Part model, mm, in its own coordinate system. A direction names the side the tool comes from. Give positions to 0.01 mm unless a question says otherwise; leave off trailing zeros. Write each loop counter-clockwise with the first axis right and the second up, starting at its lowest first coordinate (ties: lowest second). Pieces come first, ordered by that corner, then holes.
from build123d import *

# Parameters (mm, degrees)
SKETCH_1_W          = 100
SKETCH_1_H          = 52
EXTRUDE_1_DEPTH     = 8.6
SKETCH_2_W          = 97
SKETCH_2_H          = 49
CUT_EXTRUDE_1_DEPTH = 3
SKETCH_3_R          = 1.1
SKETCH_3_W          = 38.632034186
SKETCH_3_H          = 7.399361665
SKETCH_3_W_2        = 5
SKETCH_3_H_2        = 5
CUT_EXTRUDE_2_DEPTH = 61.603041755
FILLET_1_R          = 2
SKETCH_4_W          = 1.5
SKETCH_4_H          = 6.8
CUT_EXTRUDE_3_DEPTH = 1
SKETCH_5_W          = 97
SKETCH_5_H          = 49
CUT_EXTRUDE_4_DEPTH = 3
EXTRUDE_2_DEPTH     = 3
FILLET_2_R          = 3
FILLET_3_R          = 2
FILLET_5_R          = 1


with BuildPart() as part:
    # 草图1 → 凸台-拉伸1 (new body)
    with BuildSketch(Plane(origin=(0, 0, 0), x_dir=(1, 0, 0), z_dir=(0, 1, 0))):
        with Locations((1.17145908, 5.982033169)):
            Rectangle(SKETCH_1_W, SKETCH_1_H)
    extrude(amount=EXTRUDE_1_DEPTH)

    # 草图2 → 切除-拉伸1 (cut)
    with BuildSketch(Plane.XZ):
        with Locations((1.17145908, -5.982033169)):
            Rectangle(SKETCH_2_W, SKETCH_2_H)
    extrude(amount=-CUT_EXTRUDE_1_DEPTH, mode=Mode.SUBTRACT)

    # 草图3 → 切除-拉伸2 (cut, through all)
    with BuildSketch(Plane.XZ.offset(-3)):
        with Locations(Location((-12.82854092, 15.517966831, 0), (0, 0, 270))):
            Circle(SKETCH_3_R)
        with Locations(Location((39.17145908, 15.517966831, 0), (0, 0, 270))):
            Circle(SKETCH_3_R)
        with Locations(Location((39.17145908, -27.482033169, 0), (0, 0, 270))):
            Circle(SKETCH_3_R)
        with Locations(Location((-12.82854092, -27.482033169, 0), (0, 0, 270))):
            Circle(SKETCH_3_R)
        with Locations((16.615396969, 13.018709543)):
            Rectangle(SKETCH_3_W, SKETCH_3_H)
        with Locations((-13.82854092, -12.482033169)):
            Rectangle(SKETCH_3_W_2, SKETCH_3_H_2)
        with Locations((23.17145908, -12.21289677)):
            Rectangle(SKETCH_3_W_2, SKETCH_3_H_2)
    extrude(amount=-CUT_EXTRUDE_2_DEPTH, mode=Mode.SUBTRACT)

    # 圆角1
    fillet_1_edges = [part.edges().sort_by_distance(p)[0] for p in [
        (20.67145908, 5.8, -14.71289677),
        (20.67145908, 5.8, -9.71289677),
        (25.67145908, 5.8, -9.71289677),
        (25.67145908, 5.8, -14.71289677),
        (-16.32854092, 5.8, -14.982033169),
        (-16.32854092, 5.8, -9.982033169),
        (-11.32854092, 5.8, -9.982033169),
        (-11.32854092, 5.8, -14.982033169),
    ]]
    fillet(fillet_1_edges, radius=FILLET_1_R)

    # 草图4 → 切除-拉伸3 (cut)
    with BuildSketch(Plane.XZ):
        with Locations((50.42145908, 0.917966831)):
            Rectangle(SKETCH_4_W, SKETCH_4_H)
    extrude(amount=-CUT_EXTRUDE_3_DEPTH, mode=Mode.SUBTRACT)

    # 草图5 → 切除-拉伸4 (cut)
    with BuildSketch(Plane(origin=(0, 8.6, 0), x_dir=(1, 0, 0), z_dir=(0, 1, 0))):
        with Locations((1.17145908, 5.982033169)):
            Rectangle(SKETCH_5_W, SKETCH_5_H)
    extrude(amount=-CUT_EXTRUDE_4_DEPTH, mode=Mode.SUBTRACT)

    # 草图7 → 凸台-拉伸2 (add, through all)
    with BuildSketch(Plane(origin=(0, 5.6, 0), x_dir=(1, 0, 0), z_dir=(0, 1, 0))):
        Polygon((-8.68854092, -18.517966831), (-8.68854092, 4.782033169), (-27.62854092, 4.782033169), (-27.62854092, 30.482033169), (-26.12854092, 30.482033169), (-26.12854092, 6.282033169), (-8.68854092, 6.282033169), (-8.68854092, 30.482033169), (-7.18854092, 30.482033169), (-7.18854092, -4.517966831), (49.67145908, -4.517966831), (49.67145908, -6.017966831), (-7.18854092, -6.017966831), (-7.18854092, -18.517966831), align=None)
        Polygon((16.97145908, 30.482033169), (16.97145908, 6.682033169), (30.17145908, 6.682033169), (30.17145908, 30.482033169), (28.67145908, 30.482033169), (28.67145908, 8.182033169), (18.47145908, 8.182033169), (18.47145908, 30.482033169), align=None)
    extrude(amount=EXTRUDE_2_DEPTH)

    # 圆角2
    fillet_2_edges = [part.edges().sort_by_distance(p)[0] for p in [
        (-48.82854092, 4.3, -31.982033169),
        (51.17145908, 4.3, -31.982033169),
        (51.17145908, 4.3, 20.017966831),
        (-48.82854092, 4.3, 20.017966831),
    ]]
    fillet(fillet_2_edges, radius=FILLET_2_R)

    # 圆角3
    fillet_3_edges = [part.edges().sort_by_distance(p)[0] for p in [
        (49.67145908, 1.5, 18.517966831),
        (49.67145908, 1.5, -30.482033169),
        (-47.32854092, 1.5, -30.482033169),
        (-47.32854092, 1.5, 18.517966831),
        (-47.32854092, 7.1, 18.517966831),
        (-47.32854092, 7.1, -30.482033169),
        (49.67145908, 7.1, -30.482033169),
        (49.67145908, 7.1, 18.517966831),
        (-8.68854092, 7.1, 18.517966831),
        (-7.18854092, 7.1, 18.517966831),
        (-7.18854092, 7.1, 6.017966831),
        (49.67145908, 7.1, 6.017966831),
        (49.67145908, 7.1, 4.517966831),
        (-7.18854092, 7.1, 4.517966831),
        (-7.18854092, 7.1, -30.482033169),
        (-8.68854092, 7.1, -30.482033169),
        (-8.68854092, 7.1, -6.282033169),
        (-26.12854092, 7.1, -6.282033169),
        (-26.12854092, 7.1, -30.482033169),
        (-27.62854092, 7.1, -30.482033169),
        (-27.62854092, 7.1, -4.782033169),
        (-8.68854092, 7.1, -4.782033169),
        (18.47145908, 7.1, -30.482033169),
        (16.97145908, 7.1, -30.482033169),
        (16.97145908, 7.1, -6.682033169),
        (30.17145908, 7.1, -6.682033169),
        (30.17145908, 7.1, -30.482033169),
        (28.67145908, 7.1, -30.482033169),
        (28.67145908, 7.1, -8.182033169),
        (18.47145908, 7.1, -8.182033169),
    ]]
    fillet(fillet_3_edges, radius=FILLET_3_R)

    # 圆角5
    fillet_5_edges = [part.edges().sort_by_distance(p)[0] for p in [
        (-2.700620124, 4.3, 16.718390375),
        (35.931414062, 4.3, 16.718390375),
        (-2.700620124, 4.3, 9.31902871),
        (35.931414062, 4.3, 9.31902871),
    ]]
    fillet(fillet_5_edges, radius=FILLET_5_R)


solid = part.part
1) Saw through at D-D (z = -18.5). Write the cut outline in (x, y), and give its area (3 significant figures).
Check result:
outline: (-48.83, 0) - (-47.33, 0) - (-47.33, 3) - (49.67, 3) - (49.67, 0) - (51.17, 0) - (51.17, 8.6) - (49.67, 8.6) - (49.67, 5.6) - (30.17, 5.6) - (30.17, 8.6) - (28.67, 8.6) - (28.67, 5.6) - (18.47, 5.6) - (18.47, 8.6) - (16.97, 8.6) - (16.97, 5.6) - (-7.19, 5.6) - (-7.19, 8.6) - (-8.69, 8.6) - (-8.69, 5.6) - (-26.13, 5.6) - (-26.13, 8.6) - (-27.63, 8.6) - (-27.63, 5.6) - (-47.33, 5.6) - (-47.33, 8.6) - (-48.83, 8.6) - close
area: 296 mm2
2) Saw through at C-C (y = 7.5). State how many separate pieces and enclosed holes the cut face has, and give its area (3 significant figures).
Check result:
separate pieces: 1
enclosed holes: 5
area: 767 mm2
3) Saw through at A-A (z = 0.5). Write the cut outline in (x, y), and give its area (3 significant figures).
Check result:
outline: (-48.83, 0) - (-47.33, 0) - (-47.33, 3) - (49.67, 3) - (49.67, 1) - (51.17, 1) - (51.17, 8.6) - (49.67, 8.6) - (49.67, 5.6) - (-7.19, 5.6) - (-7.19, 8.6) - (-8.69, 8.6) - (-8.69, 5.6) - (-47.33, 5.6) - (-47.33, 8.6) - (-48.83, 8.6) - close
area: 281 mm2
4) Saw through at B-B (x = -20.5). Write the cut outline in (y, z).
Check result:
outline: (0, -31.98) - (8.6, -31.98) - (8.6, -30.48) - (5.6, -30.48) - (5.6, -6.28) - (8.6, -6.28) - (8.6, -4.78) - (5.6, -4.78) - (5.6, 18.52) - (8.6, 18.52) - (8.6, 20.02) - (0, 20.02) - (0, 18.52) - (3, 18.52) - (3, -30.48) - (0, -30.48) - close
5) Mould opens along Z. For faces 1 (the cylindrical face through (28.1, 7.12, -8.78)), 2 (the cylindrical face through (50.27, 4.36, 19.16)), 3 (the flat face through (1, 4, -31.982)) say: +Z half, -Z half, draft (parallel to the pull), parting line (faces both ways), or undercut.
Check result:
face 1: undercut
face 2: +Z half
face 3: -Z half
6) Drill centre lines: L1, parallel to X at y = 7.25, z = 13; L2, parallel to Z at x = 5.5, y = 7; L3, parallel to Z at x = 19.5, y = 4.5. Where is each one in solid material? Low to high.
Check result:
L1: x = -48.83 to -47.33, -8.69 to -7.19, 49.67 to 51.17
L2: z = -31.98 to -30.48, 4.52 to 6.02, 18.52 to 20.02
L3: z = -31.98 to 9.32, 16.72 to 20.02
7) Flat gauge pins, fed straight in: P1, Ø6, axis at x = 20.5, z = -18, coming from the -Y side; P2, Ø1.2, axis at x = 50.5, z = 2, coming from the -Y side; P3, Ø3, axis at x = 39.17, z = 15.52, coming from the +Y side. Where does each tip first touch, or does it go through?
Check result:
P1: stops at y = 3
P2: stops at y = 1
P3: stops at y = 5.6
8) 3-axis set-ups, long thin cutter, end or side, ignore diameter. For faces 4 (the flat face through (21, 5.6, 8)), 5 (the flat face through (49.671, 1, -6)): which of +Z, -Z, +X, -X, +Y, -Y reach the whole face in a straight line?
Check result:
face 4: +Y
face 5: -Y
